The listing builds one solid part. Answer for the finished solid, in the listing's coordinates (mm). A direction names the side the tool comes from. Coordinates: 2 decimals unless noted, no trailing zeros. Loops run counter-clockwise (first coordinate to the right, second up) from the corner with the lowest first, then second, coordinate; pieces in that order, holes last. Notation, with made-up numbers: M 43,-18.5 L 70,-18.5 A15 cw 70,-3.5 Z; hole C 29,24 d6. An arc over 180 degrees is marked long. Answer as a JSON object with one key per item and string values. Group by question number.
1. Given pin 1 (4 mm diameter, centred on x = 72.5, y = 1.5, fed in from -Z); pin 2 (5 mm diameter, centred on x = 125.5, z = -94.5, fed in from +Y); pin 3 (5.5 mm diameter, centred on y = 2, z = -130.5, fed in from -X), each flat-ended and moving along its own axis, determine where each tip first touches the part or whether it passes through.
2. A cutting plane is placed at C-C on y = 25.5. Give the vertices of the cut face in (x, z).
3. A cutting plane is placed at B-B on x = 70. Give the vertices of the cut face in (y, z).
4. A cutting plane is placed at D-D on z = -92.5. Give the vertices of the cut face in (x, y), and give its area (4 significant figures).
5. Determine the mould class of faces 1 (the face through (122, 2, -10)), 2 (the face through (25, 2, -133)), 3 (the face through (138, 3, -74)), 4 (the face through (0, 25, -74)) for opening direction X: released by +X, released by -X, zero draft, split by the parting line, or undercut.
6. A cutting plane is placed at A-A on z = -33.5. Give the vertices of the cut face in (x, y).
7. Straight lines are drawn through the part: L1, parallel to X at y = 20, z = -31; L2, parallel to Z at x = 9, y = 18; L3, parallel to X at y = 8.75, z = -111.5. For each, find the intervals that lie inside material, in ascending order.
8. For faces 5 (the face through (70, 7, -50)), 6 (the face through (122, 2, -125)), 7 (the face through (3, 2, -74)), determine the directions among +Z, -Z, +X, -X, +Y, -Y from which every point of the face is accessible in a straight line to the end or side of a thin tool.
from build123d import *

# Parameters (mm, degrees)
SKETCH3_W           = 140
SKETCH3_H           = 150
BOSS_EXTRUDE1_DEPTH = 15
SKETCH19_W          = 15
SKETCH19_H          = 15
CUT_EXTRUDE1_DEPTH  = 5
SKETCH20_W          = 15
SKETCH20_H          = 15
CUT_EXTRUDE2_DEPTH  = 5
SKETCH21_W          = 15
SKETCH21_H          = 15
CUT_EXTRUDE3_DEPTH  = 5
SKETCH22_W          = 15
SKETCH22_H          = 15
CUT_EXTRUDE4_DEPTH  = 5
SKETCH24_W          = 20
SKETCH24_H          = 20
CUT_EXTRUDE6_DEPTH  = 5
SKETCH25_R          = 4
CUT_EXTRUDE7_DEPTH  = 206.730406114
SKETCH26_W          = 10
SKETCH26_H          = 20
CUT_EXTRUDE8_DEPTH  = 206.730406114
SKETCH27_W          = 5
SKETCH27_H          = 150
BOSS_EXTRUDE2_DEPTH = 30
SKETCH28_W          = 135
SKETCH28_H          = 5
BOSS_EXTRUDE3_DEPTH = 30
SKETCH29_W          = 5
SKETCH29_H          = 145
BOSS_EXTRUDE4_DEPTH = 30
SKETCH30_W          = 130
SKETCH30_H          = 5
BOSS_EXTRUDE5_DEPTH = 30
CHAMFER2_SIZE       = 5


with BuildPart() as part:
    # Sketch3 → Boss-Extrude1 (new body)
    with BuildSketch(Plane(origin=(0, 0, 0), x_dir=(1, 0, 0), z_dir=(0, 1, 0))):
        with Locations((70, 75)):
            Rectangle(SKETCH3_W, SKETCH3_H)
    extrude(amount=BOSS_EXTRUDE1_DEPTH)

    # Sketch19 → Cut-Extrude1 (cut)
    with BuildSketch(Plane.XZ):
        with Locations((17.5, -17.5)):
            Rectangle(SKETCH19_W, SKETCH19_H)
    extrude(amount=-CUT_EXTRUDE1_DEPTH, mode=Mode.SUBTRACT)

    # Sketch20 → Cut-Extrude2 (cut)
    with BuildSketch(Plane.XZ):
        with Locations((122.5, -17.5)):
            Rectangle(SKETCH20_W, SKETCH20_H)
    extrude(amount=-CUT_EXTRUDE2_DEPTH, mode=Mode.SUBTRACT)

    # Sketch21 → Cut-Extrude3 (cut)
    with BuildSketch(Plane.XZ):
        with Locations((17.5, -132.5)):
            Rectangle(SKETCH21_W, SKETCH21_H)
    extrude(amount=-CUT_EXTRUDE3_DEPTH, mode=Mode.SUBTRACT)

    # Sketch22 → Cut-Extrude4 (cut)
    with BuildSketch(Plane.XZ):
        with Locations((122.5, -132.5)):
            Rectangle(SKETCH22_W, SKETCH22_H)
    extrude(amount=-CUT_EXTRUDE4_DEPTH, mode=Mode.SUBTRACT)

    # Sketch24 → Cut-Extrude6 (cut)
    with BuildSketch(Plane.XZ):
        with Locations((70, -75)):
            Rectangle(SKETCH24_W, SKETCH24_H)
    extrude(amount=-CUT_EXTRUDE6_DEPTH, mode=Mode.SUBTRACT)

    # Sketch25 → Cut-Extrude7 (cut, through all)
    with BuildSketch(Plane(origin=(0, 0, 0), x_dir=(-1, 0, 0), z_dir=(0, -1, 0))):
        with Locations(Location((-70, 111.5, 0), (0, 0, 90))):
            Circle(SKETCH25_R)
    extrude(amount=-CUT_EXTRUDE7_DEPTH, mode=Mode.SUBTRACT)

    # Sketch26 → Cut-Extrude8 (cut, through all)
    with BuildSketch(Plane.XZ):
        with Locations((70, -40)):
            Rectangle(SKETCH26_W, SKETCH26_H)
    extrude(amount=-CUT_EXTRUDE8_DEPTH, mode=Mode.SUBTRACT)

    # Sketch27 → Boss-Extrude2 (add)
    with BuildSketch(Plane(origin=(0, 15, 0), x_dir=(1, 0, 0), z_dir=(0, 1, 0))):
        with Locations((2.5, 75)):
            Rectangle(SKETCH27_W, SKETCH27_H)
    extrude(amount=BOSS_EXTRUDE2_DEPTH)

    # Sketch28 → Boss-Extrude3 (add)
    with BuildSketch(Plane(origin=(0, 15, 0), x_dir=(1, 0, 0), z_dir=(0, 1, 0))):
        with Locations((72.5, 147.5)):
            Rectangle(SKETCH28_W, SKETCH28_H)
    extrude(amount=BOSS_EXTRUDE3_DEPTH)

    # Sketch29 → Boss-Extrude4 (add)
    with BuildSketch(Plane(origin=(0, 15, 0), x_dir=(1, 0, 0), z_dir=(0, 1, 0))):
        with Locations((137.5, 72.5)):
            Rectangle(SKETCH29_W, SKETCH29_H)
    extrude(amount=BOSS_EXTRUDE4_DEPTH)

    # Sketch30 → Boss-Extrude5 (add)
    with BuildSketch(Plane(origin=(0, 15, 0), x_dir=(1, 0, 0), z_dir=(0, 1, 0))):
        with Locations((70, 2.5)):
            Rectangle(SKETCH30_W, SKETCH30_H)
    extrude(amount=BOSS_EXTRUDE5_DEPTH)

    # Chamfer2
    chamfer2_edges = [part.edges().sort_by_distance(p)[0] for p in [
        (70, 0, 0),
        (140, 0, -75),
        (70, 0, -150),
        (0, 0, -75),
    ]]
    chamfer(chamfer2_edges, length=CHAMFER2_SIZE)


solid = part.part
From the geometry:
{
 "1": {"pin 1": "stops at z = -148.5", "pin 2": "stops at y = 15", "pin 3": "stops at x = 0.25"},
 "2": {"outline": "M 0,-150 L 140,-150 L 140,0 L 0,0 Z; hole M 5,-145 L 135,-145 L 135,-5 L 5,-5 Z"},
 "3": {"outline": "M 0,-145 L 5,-150 L 45,-150 L 45,-145 L 15,-145 L 15,-115.5 L 0,-115.5 Z; M 0,-107.5 L 15,-107.5 L 15,-50 L 0,-50 L 0,-65 L 5,-65 L 5,-85 L 0,-85 Z; M 0,-30 L 15,-30 L 15,-5 L 45,-5 L 45,0 L 5,0 L 0,-5 Z"},
 "4": {"outline": "M 0,5 L 5,0 L 135,0 L 140,5 L 140,45 L 135,45 L 135,15 L 5,15 L 5,45 L 0,45 Z", "area": "2,375 mm²"},
 "5": {"face 1": "undercut", "face 2": "undercut", "face 3": "released by +X", "face 4": "released by -X"},
 "6": {"outline": "M 0,5 L 5,0 L 65,0 L 65,15 L 5,15 L 5,45 L 0,45 Z; M 75,0 L 135,0 L 140,5 L 140,45 L 135,45 L 135,15 L 75,15 Z"},
 "7": {"L1": "x = 0 to 5, 135 to 140", "L2": "z = -150 to -145, -5 to 0", "L3": "x = 0 to 66, 74 to 140"},
 "8": {"face 5": "+Y, -Y", "face 6": "-Y", "face 7": "+Z, -Z, -X, -Y"}
}
